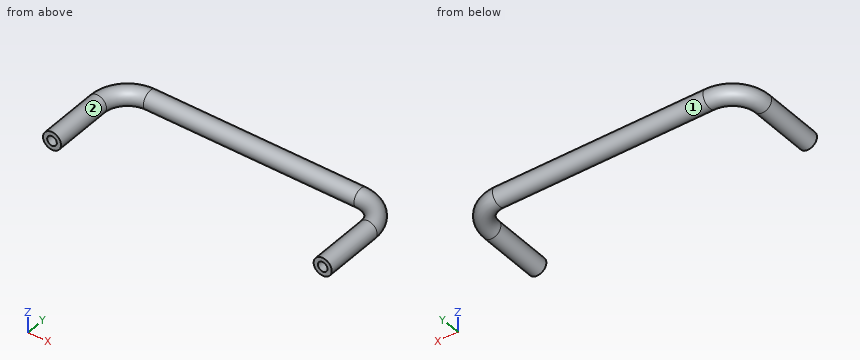
from build123d import *

# Parameters (mm, degrees)
SKETCH_2_R          = 3
SKETCH_3_R          = 1.6
CUT_EXTRUDE_1_DEPTH = 10


with BuildPart() as part:
    # 扫描1: sweep along a path in 草图1
    with BuildLine(Plane.XY) as sweep_1_path:
        Line((0, 0), (0, 20))
        ThreePointArc((0, 20), (2.928932188, 27.071067812), (10, 30))
        Line((10, 30), (80, 30))
        ThreePointArc((80, 30), (87.071067812, 27.071067812), (90, 20))
        Line((90, 20), (90, 0))
    # 草图2 → 扫描1 (sweep)
    with BuildSketch(Plane(origin=(0, 0, 0), x_dir=(1, 0, 0), z_dir=(0, 1, 0))):
        Circle(SKETCH_2_R)
    sweep(path=sweep_1_path.line)

    # 草图3 → 切除-拉伸1 (cut)
    with BuildSketch(Plane.XZ):
        with Locations(Location((0, 0, 0), (0, 0, 270))):
            Circle(SKETCH_3_R)
        with Locations(Location((90, 0, 0), (0, 0, 270))):
            Circle(SKETCH_3_R)
    extrude(amount=-CUT_EXTRUDE_1_DEPTH, mode=Mode.SUBTRACT)


solid = part.part
Input: part model. Units: mm. Frame: model coordinates. Face numbers are marked on the shaded views. A direction names the side the tool comes from. Coordinates: 2 decimals unless noted, no trailing zeros. Loops run counter-clockwise (first coordinate to the right, second up) from the corner with the lowest first, then second, coordinate; pieces in that order, holes last. Notation, with made-up numbers: (54, -32.5) -> (76, -32.5) arc R21 ccw to (76, -14.5) -> close; hole circle Ø10 at (31, -18.5). An arc over 180 degrees is marked (long way). Write each question's results on one line, items separated by ' | '. Start each with the question number.
Q1. Pin query (flat end, axial travel): pin 1 (1 mm diameter, centred on x = 53.5, z = 0.5, fed in from -Y); pin 2 (4 mm diameter, centred on x = 81.5, y = 26.5, fed in from -Z); pin 3 (3 mm diameter, centred on x = 0, z = 0, fed in from +Y); pin 4 (10 mm diameter, centred on x = 35, y = 18, fed in from -Z). Return the tip coordinate at first contact, or that it passes through.
Q2. Reachability of the marked faces 1 and 2 from +Z, -Z, +X, -X, +Y, -Y: full face, straight path, thin tool, end or side. Return the list, or none.
Q3. Section A-A, the plane y = 13. Return the cut outline in (x, z), plus the area to 3 significant figures.
Q4. Section C-C, the plane x = 56. Return the cut outline in (y, z).
Q5. Section B-B, the plane z = 0. Return the cut outline in (x, y), plus the area to 3 significant figures.
Q6. Ray query, line 1 (X direction, y = 5, z = 0); line 2 (X direction, y = 9, z = -1); line 3 (X direction, y = 8, z = 2). Return the intervals inside material, ascending. Write a range as from..to.
Found:
1) pin 1: y = 27 | pin 2: z = -2.69 | pin 3: y = 29.84 | pin 4: through
2) face 1: none | face 2: -Y
3) outline: circle Ø6 at (0, 0); circle Ø6 at (90, 0) | area: 56.5 mm2
4) outline: circle Ø6 at (30, 0)
5) outline: (-3, 0) -> (-1.6, 0) -> (-1.6, 10) -> (1.6, 10) -> (1.6, 0) -> (3, 0) -> (3, 20) arc R7 cw to (10, 27) -> (80, 27) arc R7 cw to (87, 20) -> (87, 0) -> (88.4, 0) -> (88.4, 10) -> (91.6, 10) -> (91.6, 0) -> (93, 0) -> (93, 20) arc R13 ccw to (80, 33) -> (10, 33) arc R13 ccw to (-3, 20) -> close | area: 784 mm2
6) line 1: -3..-1.6, 1.6..3, 87..88.4, 91.6..93 | line 2: -2.83..-1.25, 1.25..2.83, 87.17..88.75, 91.25..92.83 | line 3: -2.24..2.24, 87.76..92.24
